Model file for the job. Use its own axes, mm. A direction names the side the tool comes from. Give positions to 0.01 mm unless a question says otherwise; leave off trailing zeros. Order: outer loops, then holes, each group sorted by start corner. A loop starts at its lowest first (then second) coordinate and runs counter-clockwise, first axis right, second up. Notation, with made-up numbers: M 82,-30 L 136,-30 A9 ccw 136,-22 Z; hole C 48.25,77 d1. An arc over 180 degrees is marked long. Return JSON: item names as keys, results as strings. Group by question number.
1. Slice it at C-C on x = -3. List the corners of the cut face in (y, z).
2. Wall check: probe 1 along X at (y, z) = (0.7, -19) (3 decimals); probe 2 along Z at (x, y) = (-0.5, 1.9); probe 3 along Z at (x, y) = (-3, 0.95). Give the ranges that are in metal, low to high. Write a range as [from, to].
3. Slice it at D-D on x = 5. List the corners of the cut face in (y, z), then the cut area to 3 significant figures.
4. Pin check, flat tips, straight feed: pin 1 (3 mm diameter, centred on x = -15.5, z = -5, fed in from -Y); pin 2 (1.5 mm diameter, centred on x = 12, y = 1.5, fed in from +Z); pin 3 (1.5 mm diameter, centred on y = 1.5, z = -30, fed in from +X); pin 4 (0.9 mm diameter, centred on y = 2, z = -30, fed in from -X). Stop position of each tip, or through.
5. 3-axis set-ups, long thin cutter, end or side, ignore diameter. For faces 1 (the face through (19, 1, -28.5)), 2 (the face through (-17.45, 1, -30)), 3 (the face through (7.375, 2, -27)): which of +Z, -Z, +X, -X, +Y, -Y reach the whole face in a straight line?
6. Slice it at B-B on z = -16. List the corners of the cut face in (x, y).
7. Two-plate mould, pull along X, no slides. Class faces 4 (the face through (-12.576, 1.479, -34.948)), 5 (the face through (-7.375, 2, -27)), 6 (the face through (0.1, 1.5, -12.5)), 7 (the face through (17.45, 1, -30)): released by +X, released by -X, zero draft, split by the parting line, or undercut.
from build123d import *

# Parameters (mm, degrees)
BOSS_EXTRUDE1_DEPTH = 3
CUT_EXTRUDE1_DEPTH  = 3
CHAMFER1_SIZE       = 1


with BuildPart() as part:
    # Sketch1 → Boss-Extrude1 (new body)
    with BuildSketch(Plane(origin=(0, 0, 0), x_dir=(1, 0, 0), z_dir=(0, 1, 0))):
        with BuildLine():
            Line((-21.15, 28.5), (-21.15, -28.5))
            ThreePointArc((-21.15, -28.5), (0, -33.5), (21.15, -28.5))
            Line((21.15, -28.5), (21.15, 28.5))
            Line((21.15, 28.5), (-21.15, 28.5))
        make_face()
        with BuildLine():
            Line((-17.45, 32), (-17.45, 28.5))
            Line((-17.45, 28.5), (17.45, 28.5))
            Line((17.45, 28.5), (17.45, 32))
            ThreePointArc((17.45, 32), (0, 37.8), (-17.45, 32))
        make_face()
    extrude(amount=BOSS_EXTRUDE1_DEPTH)

    # Sketch2 → Cut-Extrude1 (cut)
    with BuildSketch(Plane(origin=(0, 3, 0), x_dir=(1, 0, 0), z_dir=(0, 1, 0))):
        with BuildLine():
            Line((-7.375, 17.3), (-7.375, 37.8))
            Line((-7.375, 37.8), (7.375, 37.8))
            Line((7.375, 37.8), (7.375, 17.3))
            ThreePointArc((7.375, 17.3), (0, 12.5), (-7.375, 17.3))
        make_face()
    extrude(amount=-CUT_EXTRUDE1_DEPTH, mode=Mode.SUBTRACT)

    # Chamfer1
    chamfer1_edges = [part.edges().sort_by_distance(p)[0] for p in [
        (21.15, 3, 0),
        (-21.15, 3, 0),
    ]]
    chamfer(chamfer1_edges, length=CHAMFER1_SIZE)


solid = part.part
Result:
{
 "1": {"outline": "M 0,-13.08 L 3,-13.08 L 3,33.4 L 0,33.4 Z"},
 "2": {"probe 1": "x = [-21.15, -7.375], [7.375, 21.15]", "probe 2": "z = [-12.52, 33.5]", "probe 3": "z = [-13.08, 33.4]"},
 "3": {"outline": "M 0,-14.24 L 3,-14.24 L 3,33.23 L 0,33.23 Z", "area": "142 mm2"},
 "4": {"pin 1": "stops at y = 0", "pin 2": "stops at z = 32.14", "pin 3": "stops at x = 17.45", "pin 4": "stops at x = -17.45"},
 "5": {"face 1": "-Z, +X, +Y, -Y", "face 2": "-Z, -X, +Y, -Y", "face 3": "-Z, +Y, -Y"},
 "6": {"outline": "M -21.15,0 L -6.65,0 L -6.65,3 L -20.15,3 L -21.15,2 Z; M 6.65,0 L 21.15,0 L 21.15,2 L 20.15,3 L 6.65,3 Z"},
 "7": {"face 4": "released by -X", "face 5": "undercut", "face 6": "undercut", "face 7": "released by +X"}
}
